For this review, use the dimensioned drawing (mm, ordinates from the lowest corner) and the shaded views. A direction names the side the tool comes from. Round coordinates to 2 decimals unless told otherwise and drop trailing zeros. Loops run counter-clockwise (first coordinate to the right, second up) from the corner with the lowest first, then second, coordinate; pieces in that order, holes last. Notation, with made-up numbers: M 4.5,-39 L 16.5,-39 A20 ccw 16.5,-4 Z; hole C 31.25,82 d6. An arc over 180 degrees is marked long. Use a Markdown table: item, result. Add a question column.
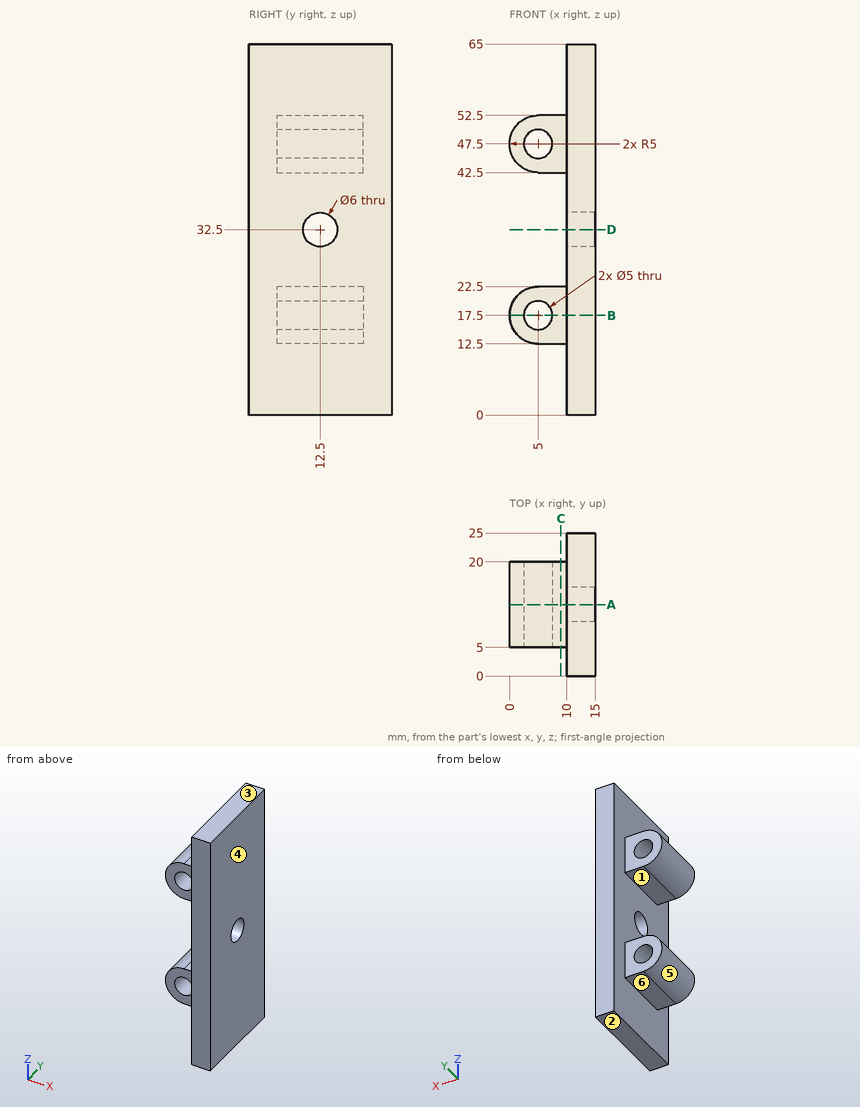
(1) To check wall thickness, follow probe 1 along Z at (x, y) = (4.75, 7.75); probe 2 along Z at (x, y) = (8.5, 9); probe 3 along Y at (x, z) = (13.9, 32.5). State the ranges of each line that lie inside material, in increasing order.
(2) Insertion check: pin 1 Ø8 at (y, z) = (12.5, 32.5) entering from -X; pin 2 Ø2.5 at (x, y) = (6.5, 15) entering from +Z; pin 3 Ø8 at (x, z) = (5.5, 18.5) entering from -Y. Each pin has a flat end and moves straight along its axis. Give the tip position at first contact, or say it passes through.
(3) Consider section D-D, the plane z = 32.5. Give the boundary of the cut face in (x, y), then the cut area to 3 significant figures.
(4) Consider section A-A, the plane y = 12.5. Give the boundary of the cut face in (x, z).
(5) Consider section C-C, the plane x = 9. Give the boundary of the cut face in (y, z).
(6) Draft analysis for pull direction Z (two halves, no side actions). For the marked faces 3, 4, 5 and 6, state which applies: released by +Z, released by -Z, zero draft, split by the parting line, or undercut.
(7) Consider section B-B, the plane z = 17.5. Give the boundary of the cut face in (x, y).
(8) For the marked faces 1 and 2, list the 3-axis set-ups (+Z, -Z, +X, -X, +Y, -Y) from which the entire face can be reached by the end or side of a thin tool; tool diameter is ignored.
Found:
| question | item | result |
|---|---|---|
| 1 | probe 1 | z = 12.51 to 15.01, 19.99 to 22.49, 42.51 to 45.01, 49.99 to 52.49 |
| 1 | probe 2 | z = 12.5 to 22.5, 42.5 to 52.5 |
| 1 | probe 3 | y = 0 to 9.5, 15.5 to 25 |
| 2 | pin 1 | stops at x = 10 |
| 2 | pin 2 | stops at z = 52.5 |
| 2 | pin 3 | stops at y = 5 |
| 3 | outline | M 10,0 L 15,0 L 15,9.5 L 10,9.5 Z; M 10,15.5 L 15,15.5 L 15,25 L 10,25 Z |
| 3 | area | 95.0 mm^2 |
| 4 | outline | M 5,12.5 L 10,12.5 L 10,0 L 15,0 L 15,29.5 L 10,29.5 L 10,22.5 L 5,22.5 A5 ccw Z; M 5,42.5 L 10,42.5 L 10,35.5 L 15,35.5 L 15,65 L 10,65 L 10,52.5 L 5,52.5 A5 ccw Z; hole C 5,17.5 d5; hole C 5,47.5 d5 |
| 5 | outline | M 5,12.5 L 20,12.5 L 20,22.5 L 5,22.5 Z; M 5,42.5 L 20,42.5 L 20,52.5 L 5,52.5 Z |
| 6 | face 3 | released by +Z |
| 6 | face 4 | zero draft |
| 6 | face 5 | undercut |
| 6 | face 6 | released by -Z |
| 7 | outline | M 0,5 L 2.5,5 L 2.5,20 L 0,20 Z; M 7.5,5 L 10,5 L 10,0 L 15,0 L 15,25 L 10,25 L 10,20 L 7.5,20 Z |
| 8 | face 1 | -X, +Y, -Y |
| 8 | face 2 | -Z, +X, -X, +Y, -Y |
